from build123d import *

# Parameters (mm, degrees)
SKETCH1_R           = 60.325
BOSS_EXTRUDE1_DEPTH = 15.748
SKETCH2_R           = 9.525
CUT_EXTRUDE1_DEPTH  = 7.62
SKETCH3_R           = 4.7625
CUT_EXTRUDE2_DEPTH  = 86.698749314
SKETCH4_R           = 25.4
BOSS_EXTRUDE2_DEPTH = 50.8
SKETCH5_R           = 17.4244
CUT_EXTRUDE3_DEPTH  = 109.198186464
CUT_EXTRUDE4_DEPTH  = 109.198186464
FILLET1_R           = 3.048


with BuildPart() as part:
    # Sketch1 → Boss-Extrude1 (new body)
    with BuildSketch(Plane(origin=(0, 0, 0), x_dir=(1, 0, 0), z_dir=(0, 1, 0))):
        with Locations(Location((0, 0, 0), (0, 0, 270))):
            Circle(SKETCH1_R)
    extrude(amount=BOSS_EXTRUDE1_DEPTH)

    # Sketch2 → Cut-Extrude1 (cut)
    with BuildSketch(Plane(origin=(0, 15.748, 0), x_dir=(1, 0, 0), z_dir=(0, 1, 0))):
        with Locations(Location((0, -42.926, 0), (0, 0, 270))):
            Circle(SKETCH2_R)
        with Locations(Location((42.926, 0, 0), (0, 0, 270))):
            Circle(SKETCH2_R)
        with Locations(Location((-42.926, 0, 0), (0, 0, 270))):
            Circle(SKETCH2_R)
    extrude(amount=-CUT_EXTRUDE1_DEPTH, mode=Mode.SUBTRACT)

    # Sketch3 → Cut-Extrude2 (cut, through all)
    with BuildSketch(Plane(origin=(0, 8.128, 0), x_dir=(1, 0, 0), z_dir=(0, 1, 0))):
        with Locations(Location((-42.926, 0, 0), (0, 0, 270))):
            Circle(SKETCH3_R)
        with Locations(Location((42.926, 0, 0), (0, 0, 270))):
            Circle(SKETCH3_R)
        with Locations(Location((0, -42.926, 0), (0, 0, 270))):
            Circle(SKETCH3_R)
    extrude(amount=-CUT_EXTRUDE2_DEPTH, mode=Mode.SUBTRACT)

    # Sketch4 → Boss-Extrude2 (add)
    with BuildSketch(Plane(origin=(0, 15.748, 0), x_dir=(1, 0, 0), z_dir=(0, 1, 0))):
        with Locations(Location((0, 0, 0), (0, 0, 270))):
            Circle(SKETCH4_R)
    extrude(amount=BOSS_EXTRUDE2_DEPTH)

    # Sketch5 → Cut-Extrude3 (cut, through all)
    with BuildSketch(Plane(origin=(0, 66.548, 0), x_dir=(1, 0, 0), z_dir=(0, 1, 0))):
        with Locations(Location((0, 0, 0), (0, 0, 270))):
            Circle(SKETCH5_R)
    extrude(amount=-CUT_EXTRUDE3_DEPTH, mode=Mode.SUBTRACT)

    # Sketch7 → Cut-Extrude4 (cut, through all)
    with BuildSketch(Plane(origin=(0, 66.548, 0), x_dir=(1, 0, 0), z_dir=(0, 1, 0))):
        with BuildLine():
            Line((-6.096, 42.926), (-6.096, 31.496))
            Line((-6.096, 31.496), (-14.224, 31.496))
            Line((-14.224, 31.496), (-14.224, 0))
            Line((-14.224, 0), (14.224, 0))
            Line((14.224, 0), (14.224, 31.496))
            Line((14.224, 31.496), (6.096, 31.496))
            Line((6.096, 31.496), (6.096, 42.926))
            ThreePointArc((6.096, 42.926), (0, 49.022), (-6.096, 42.926))
        make_face()
    extrude(amount=-CUT_EXTRUDE4_DEPTH, mode=Mode.SUBTRACT)

    # Fillet1
    fillet1_edges = [part.edges().sort_by_distance(p)[0] for p in [
        (14.224, 7.874, -31.496),
        (-14.224, 7.874, -31.496),
    ]]
    fillet(fillet1_edges, radius=FILLET1_R)


solid = part.part
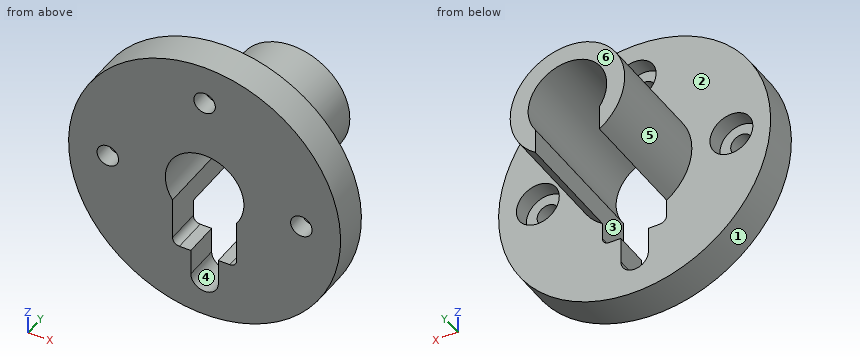
The listing builds one solid part. Answer for the finished solid, in the listing's coordinates (mm). Face numbers are marked on the shaded views. A direction names the side the tool comes from. Coordinates: 2 decimals unless noted, no trailing zeros. Write each loop counter-clockwise with the first axis right and the second up, starting at its lowest first coordinate (ties: lowest second). Pieces come first, ordered by that corner, then holes. Notation, with made-up numbers: M -37.75,-35.75 L 11.25,-35.75 A24 cw 11.25,2.25 Z; hole C 48.5,81 d2. An arc over 180 degrees is marked long. Put each result on its own line as item: value. Start each with the question number.
1. Flat-ended cylindrical pins translate along their axes: P1, Ø8, axis at x = 2, y = 49, coming from the +Z side; P2, Ø5.5, axis at x = -8, y = 11, coming from the +Z side; P3, Ø25, axis at x = 0, z = 42.926, coming from the +Y side. Find the tip coordinate at first contact, or state that the pin passes through.
2. A cutting plane is placed at B-B on x = 0. Write down the section's boundary in (y, z) (1 decimal).
3. Consider line 1 (X direction, y = 3, z = 0) (1 decimal); line 2 (X direction, y = 14, z = 0) (3 decimals); line 3 (Y direction, x = -27, z = -41). Determine where each line is inside the solid, lowest interval first. Write a range as from..to.
4. Which of the six approach directions +Z, -Z, +X, -X, +Y, -Y give full straight-line access (tool end or side, diameter ignored) to the marked faces 4, 5 and 6?
5. A cutting plane is placed at A-A on z = 0. Write down the section's boundary in (x, y) (1 decimal).
6. For a pull along Z with two mould halves and no side action, classify the marked faces 1, 2 and 3 as pulls with the +Z half, pulls with the -Z half, needs draft (parallel to the pull), parting line crosses it, or undercut.
7. A cutting plane is placed at D-D on z = -34. Write down the section's boundary in (x, y).
8. A cutting plane is placed at C-C on x = 40. Write down the section's boundary in (y, z), then the cut area to 3 significant figures.
Resolved:
1. P1: stops at z = 25.4
1. P2: stops at z = 60.1
1. P3: stops at y = 15.75
2. outline: M 0,-60.3 L 15.7,-60.3 L 15.7,-49 L 0,-49 Z; M 0,17.4 L 66.5,17.4 L 66.5,25.4 L 15.7,25.4 L 15.7,33.4 L 8.1,33.4 L 8.1,38.2 L 0,38.2 Z; M 0,47.7 L 8.1,47.7 L 8.1,52.5 L 15.7,52.5 L 15.7,60.3 L 0,60.3 Z
3. line 1: x = -60.3..-47.7, -38.2..-17.4, 17.4..38.2, 47.7..60.3
3. line 2: x = -60.325..-52.451, -33.401..-17.424, 17.424..33.401, 52.451..60.325
3. line 3: y = 0..15.75
4. face 4: +Y, -Y
4. face 5: +Y
4. face 6: +Z, -Z, +X, -X, +Y
5. outline: M -60.3,0 L -47.7,0 L -47.7,8.1 L -52.5,8.1 L -52.5,15.7 L -60.3,15.7 Z; M -38.2,0 L -17.4,0 L -17.4,66.5 L -25.4,66.5 L -25.4,15.7 L -33.4,15.7 L -33.4,8.1 L -38.2,8.1 Z; M 17.4,0 L 38.2,0 L 38.2,8.1 L 33.4,8.1 L 33.4,15.7 L 25.4,15.7 L 25.4,66.5 L 17.4,66.5 Z; M 47.7,0 L 60.3,0 L 60.3,15.7 L 52.5,15.7 L 52.5,8.1 L 47.7,8.1 Z
6. face 1: parting line crosses it
6. face 2: needs draft
6. face 3: undercut
7. outline: M -49.83,0 L -6.1,0 L -6.1,15.75 L -49.83,15.75 Z; M 6.1,0 L 49.83,0 L 49.83,15.75 L 6.1,15.75 Z
8. outline: M 0,-45.16 L 15.75,-45.16 L 15.75,-9.06 L 8.13,-9.06 L 8.13,-3.76 L 0,-3.76 Z; M 0,3.76 L 8.13,3.76 L 8.13,9.06 L 15.75,9.06 L 15.75,45.16 L 0,45.16 Z
8. area: 1,220 mm2
